```python
from build123d import *

# Parameters (mm, degrees)
ESQUISSE1_W        = 100
ESQUISSE1_H        = 12
BOSS_EXTRU_1_DEPTH = 5
BOSS_EXTRU_2_DEPTH = 4
BOSS_EXTRU_3_DEPTH = 4


with BuildPart() as part:
    # Esquisse1 → Boss.-Extru.1 (new body)
    with BuildSketch(Plane.XY):
        Rectangle(ESQUISSE1_W, ESQUISSE1_H)
    extrude(amount=BOSS_EXTRU_1_DEPTH)

    # Esquisse2 → Boss.-Extru.2 (add)
    with BuildSketch(Plane.XY.offset(5)):
        Polygon((-50, 3), (45, 3), (45, -3), (-50, -3), (-50, -6), (50, -6), (50, 6), (-50, 6), align=None)
    extrude(amount=BOSS_EXTRU_2_DEPTH)

    # Esquisse3 → Boss.-Extru.3 (add)
    with BuildSketch(Plane(origin=(0, 0, 0), x_dir=(-1, 0, 0), z_dir=(0, 0, -1))):
        Polygon((-50, -6), (50, -6), (50, -3), (-45, -3), (-45, 3), (50, 3), (50, 6), (-50, 6), align=None)
    extrude(amount=BOSS_EXTRU_3_DEPTH)


solid = part.part
```
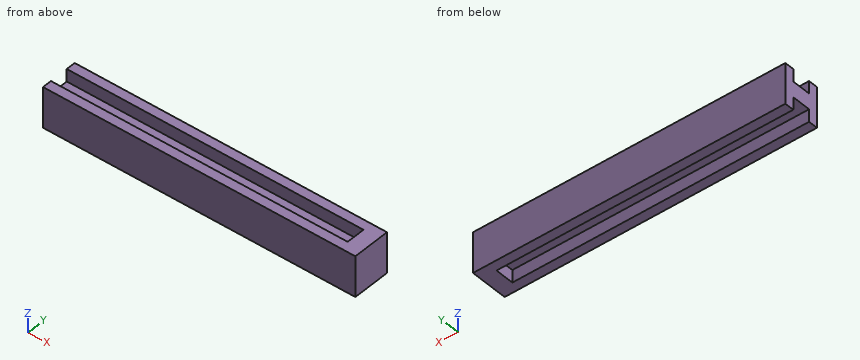
Here's how the part is built. I have some questions about the finished solid (model axes, mm). Give positions to 0.01 mm unless a question says otherwise; leave off trailing zeros. Order: outer loops, then holes, each group sorted by start corner. A loop starts at its lowest first (then second) coordinate and runs counter-clockwise, first axis right, second up. Notation, with made-up numbers: (38.25, 15.5) - (57.25, 15.5) arc R18 ccw to (57.25, 23.5) - close; hole circle Ø10 at (-19.75, 23.5). An arc over 180 degrees is marked (long way). Answer as a JSON object with one key per item and string values. Group by question number.
Item 1: For P1, Ø6.5, axis at x = -8.5, y = 1.5, coming from the -Z side; P2, Ø1, axis at x = 30.5, y = 0.5, coming from the +Z side, each with a flat end and sliding along its axis, tell me the tip position at first contact or that it passes through.
Item 2: If we section it at C-C on z = -1.25: Please give me the cut outline in (x, y).
Item 3: If we section it at A-A on x = 36.5: Please give me the cut outline in (y, z).
Item 4: If we section it at B-B on y = 1: Please give me the cut outline in (x, z), and give its area (3 significant figures).
Item 5: Please list where these lines run through material, in increasing order: probe 1 along Y at (x, z) = (-15.5, 5.5); probe 2 along Z at (x, y) = (7, 1.5); probe 3 along X at (y, z) = (0.75, -1.25).
Result set:
{
 "1": {"P1": "z = -4", "P2": "z = 5"},
 "2": {"outline": "(-50, -6) - (50, -6) - (50, 6) - (-50, 6) - (-50, 3) - (45, 3) - (45, -3) - (-50, -3) - close"},
 "3": {"outline": "(-6, -4) - (-3, -4) - (-3, 0) - (3, 0) - (3, -4) - (6, -4) - (6, 9) - (3, 9) - (3, 5) - (-3, 5) - (-3, 9) - (-6, 9) - close"},
 "4": {"outline": "(-50, 0) - (45, 0) - (45, -4) - (50, -4) - (50, 9) - (45, 9) - (45, 5) - (-50, 5) - close", "area": "540 mm²"},
 "5": {"probe 1": "-6 to -3, 3 to 6", "probe 2": "0 to 5", "probe 3": "45 to 50"}
}
